The model under review builds one solid part; all positions refer to its coordinate system, in mm. Give positions to 0.01 mm unless a question says otherwise; leave off trailing zeros. Order: outer loops, then holes, each group sorted by start corner. A loop starts at its lowest first (then second) coordinate and runs counter-clockwise, first axis right, second up. Notation, with made-up numbers: M -3.75,20 L 25.25,20 A34 ccw 25.25,54 Z; hole C -9,-9 d10. An arc over 180 degrees is marked long. One line per question, with ' | ' between items. Start each with the question number.
1. Insertion check: P1, Ø4, axis at y = 119.5, z = -7, coming from the -X side; P2, Ø1.5, axis at x = 117, z = -6.5, coming from the +Y side; P3, Ø1, axis at y = 87, z = -5.5, coming from the -X side. Each pin has a flat end and moves straight along its axis. Give the tip position at first contact, or say it passes through.
2. Wall thickness on L1, parallel to X at y = 70.5, z = -5.5; L2, parallel to X at y = 85.5, z = -6.5; L3, parallel to Y at x = -28, z = -3.25: over which ranges is each line inside the solid? List them lowest first.
3. We need section A-A on z = -6.5. Write out the cut boundary in (x, y).
4. The part is to be moulded in two halves that separate along X. For faces 1 (the face through (61.77, 110.7, -6.32)), 2 (the face through (74.7, 125.1, -1.5)), 3 (the face through (76.1, 127.5, -6.2)), say which applies: +X half, -X half, draft (parallel to the pull), parting line (faces both ways), or undercut.
Solid Edge part; units mm, degrees
sketch "Sketch1" plane through (0, 0, 0) normal (0, -1, 0) x (1, 0, 0)
  line L0 (129.7661, -1.5) -> (126.7661, -1.5)
  line L1 (126.7661, -1.5) -> (126.7661, -11)
  line L2 (126.7661, -11) -> (148.4823, -11)
  line L3 (148.4823, -11) -> (148.4823, -1.5)
  line L4 (148.4823, -1.5) -> (145.4823, -1.5)
  arc A0 (145.4823, -1.5) -> (129.7661, -1.5) centre (137.6242, 0) cw
  dimension "D1" = 129.7661
  dimension "D2" = 148.4823
revolve "RevolvedProtrusion_2" add sketch "Sketch1" angle 120 about axis through (0, 0, 0) along (0, 0, 1)
properties material "ABS Plastic, high impact"
Entries:
1) P1: stops at x = -70.1 | P2: stops at y = 92.37 | P3: stops at x = 91.72
2) L1: x = 105.35 to 111.38, 124.91 to 130.68 | L2: x = 93.59 to 101.82, 113.73 to 121.39 | L3: y = 123.64 to 127.27, 142.2 to 145.82
3) outline: M -74.24,128.59 L -71.14,123.22 A142.29 cw 142.29,0 L 148.48,0 A148.48 ccw Z; M -66.48,115.15 L -63.38,109.78 A126.77 cw 126.77,0 L 132.96,0 A132.96 ccw Z
4) face 1: undercut | face 2: draft | face 3: parting line
